from build123d import *

# Parameters (mm, degrees)
BOSS_EXTRUDE1_DEPTH      = 60
BOSS_EXTRUDE1_DEPTH_BACK = 60
SKETCH2_W                = 17.261807542
SKETCH2_H                = 108.92334372
SKETCH3_R                = 3
SKETCH3_R_2              = 1
BOSS_EXTRUDE2_DEPTH      = 5
SKETCH4_R                = 3.25
CUT_EXTRUDE1_DEPTH       = 21
CUT_EXTRUDE2_DEPTH       = 114.240882246
FILLET1_R                = 40
FILLET3_R                = 5
FILLET4_R                = 10
SKETCH6_R                = 1
CUT_EXTRUDE3_DEPTH       = 7.5
CHAMFER2_SIZE            = 2.5
CHAMFER4_SIZE            = 5
SKETCH7_R                = 1.25
CUT_EXTRUDE4_DEPTH       = 7.5


with BuildPart() as part:
    # Sketch2 → Boss-Extrude1 (new, two sides: drawn at the far end of the back side and taken through both)
    with BuildSketch(Plane.XY.offset(-BOSS_EXTRUDE1_DEPTH_BACK)):
        Polygon((-8.630903771, 54.46167186), (8.630903771, 54.46167186), (25.625086391, 54.46167186), (25.625086391, 67.842918018), (-25.625086391, 67.842918018), (-25.625086391, 54.46167186), align=None)
        Rectangle(SKETCH2_W, SKETCH2_H)
        Polygon((59.345826708, -54.46167186), (8.630903771, -54.46167186), (-8.630903771, -54.46167186), (-59.345826708, -54.46167186), (-59.345826708, -66.772418325), (59.345826708, -66.772418325), align=None)
    extrude(amount=BOSS_EXTRUDE1_DEPTH + BOSS_EXTRUDE1_DEPTH_BACK)

    # Sketch3 → Boss-Extrude2 (add)
    # profile 1 of 6: a face of its own
    with BuildSketch(Plane(origin=(8.630903771, 0, 0), x_dir=(0, 0, -1), z_dir=(1, 0, 0))):
        with Locations(Location((-6.9, 47.168726105, 0), (0, 0, 180))):
            Circle(SKETCH3_R)
        with Locations((-6.9, 47.168726105)):
            Circle(SKETCH3_R_2, mode=Mode.SUBTRACT)
    # profile 2 of 6: a face of its own
    with BuildSketch(Plane(origin=(8.630903771, 0, 0), x_dir=(0, 0, -1), z_dir=(1, 0, 0))):
        with Locations(Location((37.6, 47.168726105, 0), (0, 0, 180))):
            Circle(SKETCH3_R)
        with Locations((37.6, 47.168726105)):
            Circle(SKETCH3_R_2, mode=Mode.SUBTRACT)
    # profile 3 of 6: a face of its own
    with BuildSketch(Plane(origin=(8.630903771, 0, 0), x_dir=(0, 0, -1), z_dir=(1, 0, 0))):
        with Locations(Location((54.1, 48.818726105, 0), (0, 0, 180))):
            Circle(SKETCH3_R)
        with Locations((54.1, 48.818726105)):
            Circle(SKETCH3_R_2, mode=Mode.SUBTRACT)
    # profile 4 of 6: a face of its own
    with BuildSketch(Plane(origin=(8.630903771, 0, 0), x_dir=(0, 0, -1), z_dir=(1, 0, 0))):
        with Locations(Location((54.1, -48.691074046, 0), (0, 0, 180))):
            Circle(SKETCH3_R)
        with Locations((54.1, -48.691074046)):
            Circle(SKETCH3_R_2, mode=Mode.SUBTRACT)
    # profile 5 of 6: a face of its own
    with BuildSketch(Plane(origin=(8.630903771, 0, 0), x_dir=(0, 0, -1), z_dir=(1, 0, 0))):
        with Locations(Location((21.1, -48.691074046, 0), (0, 0, 180))):
            Circle(SKETCH3_R)
        with Locations((21.1, -48.691074046)):
            Circle(SKETCH3_R_2, mode=Mode.SUBTRACT)
    # profile 6 of 6: a face of its own
    with BuildSketch(Plane(origin=(8.630903771, 0, 0), x_dir=(0, 0, -1), z_dir=(1, 0, 0))):
        with Locations(Location((-6.9, -48.691074046, 0), (0, 0, 180))):
            Circle(SKETCH3_R)
        with Locations((-6.9, -48.691074046)):
            Circle(SKETCH3_R_2, mode=Mode.SUBTRACT)
    extrude(amount=BOSS_EXTRUDE2_DEPTH)

    # Sketch4 → Cut-Extrude1 (cut, symmetric)
    with BuildSketch(Plane(origin=(8.630903771, 0, 0), x_dir=(0, 0, -1), z_dir=(1, 0, 0))):
        with Locations((20.75, 27.46167186)):
            Circle(SKETCH4_R)
        with Locations((20.75, -27.53832814)):
            Circle(SKETCH4_R)
    extrude(amount=CUT_EXTRUDE1_DEPTH, both=True, mode=Mode.SUBTRACT)

    # Sketch5 → Cut-Extrude2 (cut, through all)
    with BuildSketch(Plane(origin=(8.630903771, 0, 0), x_dir=(0, 0, -1), z_dir=(1, 0, 0))):
        with BuildLine():
            Line((-20, 35), (-20, -35))
            ThreePointArc((-20, -35), (-35, -50), (-50, -35))
            Line((-50, -35), (-50, 35))
            ThreePointArc((-50, 35), (-35, 50), (-20, 35))
        make_face()
    extrude(amount=-CUT_EXTRUDE2_DEPTH, mode=Mode.SUBTRACT)

    # Fillet1
    fillet1_edges = [part.edges().sort_by_distance(p)[0] for p in [
        (-59.345826708, -60.617045093, -60),
        (59.345826708, -60.617045093, -60),
    ]]
    fillet(fillet1_edges, radius=FILLET1_R)

    # Fillet3
    fillet3_edges = [part.edges().sort_by_distance(p)[0] for p in [
        (-8.630903771, 0, 50),
        (-8.630903771, -50, 35),
        (-8.630903771, 0, 20),
        (-8.630903771, 50, 35),
        (8.630903771, 0, 20),
        (8.630903771, 50, 35),
        (8.630903771, 0, 50),
        (8.630903771, -50, 35),
    ]]
    fillet(fillet3_edges, radius=FILLET3_R)

    # Fillet4
    fillet4_edges = [part.edges().sort_by_distance(p)[0] for p in [
        (-25.625086391, 61.152294939, -60),
        (25.625086391, 61.152294939, -60),
    ]]
    fillet(fillet4_edges, radius=FILLET4_R)

    # Sketch6 → Cut-Extrude3 (cut)
    with BuildSketch(Plane(origin=(0, 0, -60), x_dir=(-1, 0, 0), z_dir=(0, 0, -1))):
        with Locations((11.75, 61.342918018)):
            Circle(SKETCH6_R)
        with Locations((-11.75, 61.342918018)):
            Circle(SKETCH6_R)
    extrude(amount=-CUT_EXTRUDE3_DEPTH, mode=Mode.SUBTRACT)

    # Chamfer2
    chamfer2_edges = [part.edges().sort_by_distance(p)[0] for p in [
        (-12.127995081, 54.46167186, -60),
        (-25.625086391, 54.46167186, 5),
        (-25.625086391, 67.842918018, 5),
        (-22.696154203, 54.46167186, -57.071067812),
        (0, 67.842918018, -60),
        (12.127995081, 54.46167186, -60),
        (25.625086391, 67.842918018, 5),
        (22.696154203, 67.842918018, -57.071067812),
        (-22.696154203, 67.842918018, -57.071067812),
        (25.625086391, 54.46167186, 5),
        (22.696154203, 54.46167186, -57.071067812),
        (25.625086391, 61.152294939, 60),
        (-25.625086391, 61.152294939, 60),
    ]]
    chamfer(chamfer2_edges, length=CHAMFER2_SIZE)

    # Chamfer4
    chamfer4_edges = [part.edges().sort_by_distance(p)[0] for p in [
        (-13.98836524, -54.46167186, -60),
        (-59.345826708, -54.46167186, 20),
        (-47.630097955, -54.46167186, -48.284271247),
        (59.345826708, -54.46167186, 20),
        (47.630097955, -54.46167186, -48.284271247),
        (13.98836524, -54.46167186, -60),
    ]]
    chamfer(chamfer4_edges, length=CHAMFER4_SIZE)

    # Sketch7 → Cut-Extrude4 (cut)
    with BuildSketch(Plane.XY.offset(60)):
        with Locations((0, 61.152294939)):
            Circle(SKETCH7_R)
    extrude(amount=-CUT_EXTRUDE4_DEPTH, mode=Mode.SUBTRACT)


solid = part.part
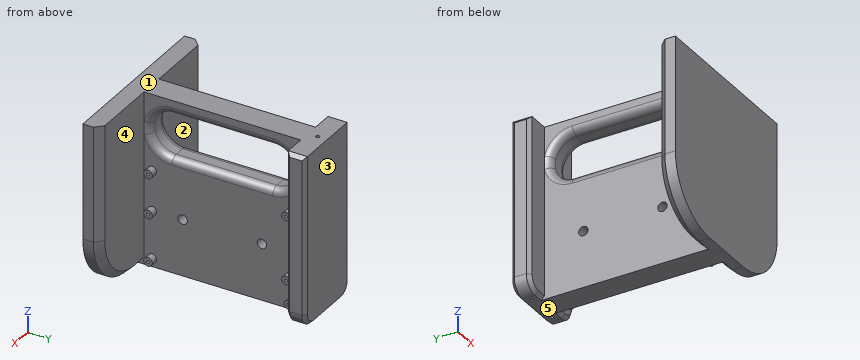
Read the model definition and answer for the solid it produces. Units are mm, in the model's axes. Face numbers are marked on the shaded views. A direction names the side the tool comes from. Give positions to 0.01 mm unless a question says otherwise; leave off trailing zeros. Write each loop counter-clockwise with the first axis right and the second up, starting at its lowest first coordinate (ties: lowest second). Pieces come first, ordered by that corner, then holes. Notation, with made-up numbers: (25, 11.5) - (82, 11.5) arc R22 ccw to (82, 46.5) - close; hole circle Ø5 at (50.25, 31). An arc over 180 degrees is marked (long way). Use CSV: the item, a comma, the result in double quotes. Start each with the question number.
(1) For the marked faces 4 and 5, determine the directions among +Z, -Z, +X, -X, +Y, -Y from which every point of the face is accessible in a straight line to the end or side of a thin tool.
(2) Determine the mould class of the marked faces 1, 2 and 3 for opening direction Y: +Y half, -Y half, draft (parallel to the pull), parting line (faces both ways), or undercut.
(3) Find section A-A (y = -9.5). Give the vertices of the cut face in (x, z).
(4) Consider line 1 along Y through (x, z) = (10.8, 6.9); line 2 along Y through (x, z) = (10.25, -37.6); line 3 along Y through (x, z) = (10, -37). Determine where each line is inside the solid, lowest interval first.
(5) Given P1, Ø5, axis at y = -17.5, z = -8.5, coming from the +X side; P2, Ø3, axis at y = 47.17, z = 6.9, coming from the +X side; P3, Ø1, axis at x = -43.5, z = -11.5, coming from the +Y side, each flat-ended and moving along its own axis, determine where each tip first touches the part or whether it passes through.
Findings below:
1,face 4,"+Z, -Z, +X"
1,face 5,"-Z, +X, -X, +Y, -Y"
2,face 1,"draft"
2,face 2,"undercut"
2,face 3,"+Y half"
3,outline,"(-8.63, -60) - (8.63, -60) - (8.63, 15) arc R5 ccw to (3.63, 20) - (-3.63, 20) arc R5 ccw to (-8.63, 15) - close; (-8.63, 55) arc R5 ccw to (-3.63, 50) - (3.63, 50) arc R5 ccw to (8.63, 55) - (8.63, 60) - (-8.63, 60) - close"
4,line 1,"-66.77 to -54.46, -51.69 to -49.69, -47.69 to -45.69, 44.17 to 46.17, 48.17 to 50.17, 54.46 to 67.84"
4,line 2,"-66.77 to -54.46, 44.17 to 46.17, 48.17 to 50.17, 54.46 to 67.84"
4,line 3,"-66.77 to -54.46, 44.23 to 46.37, 47.97 to 50.11, 54.46 to 67.84"
5,P1,"x = 8.63"
5,P2,"x = 13.63"
5,P3,"y = -54.46"
